from build123d import *

# Parameters (mm, degrees)
BOSS_EXTRUDE1_DEPTH = 150
SKETCH2_R           = 4.5
CUT_EXTRUDE2_DEPTH  = 12.5
SKETCH3_R           = 9.5
BOSS_EXTRUDE2_DEPTH = 55.5
SKETCH4_R           = 27.75
BOSS_EXTRUDE3_DEPTH = 2
SKETCH5_W           = 6
SKETCH5_H           = 35
BOSS_EXTRUDE4_DEPTH = 12


with BuildPart() as part:
    # Sketch1 → Boss-Extrude1 (new body)
    with BuildSketch(Plane(origin=(0, 0, 0), x_dir=(1, 0, 0), z_dir=(0, 1, 0))):
        with BuildLine():
            Line((-44.5, 55), (44.5, 55))
            ThreePointArc((44.5, 55), (51.924621202, 51.924621202), (55, 44.5))
            Line((55, 44.5), (55, -44.5))
            ThreePointArc((55, -44.5), (51.924621202, -51.924621202), (44.5, -55))
            Line((44.5, -55), (-44.5, -55))
            ThreePointArc((-44.5, -55), (-51.924621202, -51.924621202), (-55, -44.5))
            Line((-55, -44.5), (-55, 44.5))
            ThreePointArc((-55, 44.5), (-51.924621202, 51.924621202), (-44.5, 55))
        make_face()
    extrude(amount=BOSS_EXTRUDE1_DEPTH)

    # Sketch2 → Cut-Extrude2 (cut)
    with BuildSketch(Plane(origin=(0, 150, 0), x_dir=(1, 0, 0), z_dir=(0, 1, 0))):
        with Locations(Location((-44.5, 44.5, 0), (0, 0, 270))):
            Circle(SKETCH2_R)
        with Locations(Location((44.5, 44.5, 0), (0, 0, 270))):
            Circle(SKETCH2_R)
        with Locations(Location((-44.5, -44.5, 0), (0, 0, 270))):
            Circle(SKETCH2_R)
        with Locations(Location((44.5, -44.5, 0), (0, 0, 270))):
            Circle(SKETCH2_R)
    extrude(amount=-CUT_EXTRUDE2_DEPTH, mode=Mode.SUBTRACT)

    # Sketch3 → Boss-Extrude2 (add)
    with BuildSketch(Plane(origin=(0, 150, 0), x_dir=(1, 0, 0), z_dir=(0, 1, 0))):
        with Locations(Location((0, 0, 0), (0, 0, 270))):
            Circle(SKETCH3_R)
    extrude(amount=BOSS_EXTRUDE2_DEPTH)

    # Sketch4 → Boss-Extrude3 (add)
    with BuildSketch(Plane(origin=(0, 150, 0), x_dir=(1, 0, 0), z_dir=(0, 1, 0))):
        with Locations(Location((0, 0, 0), (0, 0, 270))):
            Circle(SKETCH4_R)
    extrude(amount=BOSS_EXTRUDE3_DEPTH)

    # Sketch5 → Boss-Extrude4 (add)
    with BuildSketch(Plane(origin=(0, 0, 0), x_dir=(0, 0, -1), z_dir=(1, 0, 0))):
        with Locations((0, 188)):
            Rectangle(SKETCH5_W, SKETCH5_H)
    extrude(amount=BOSS_EXTRUDE4_DEPTH)


solid = part.part
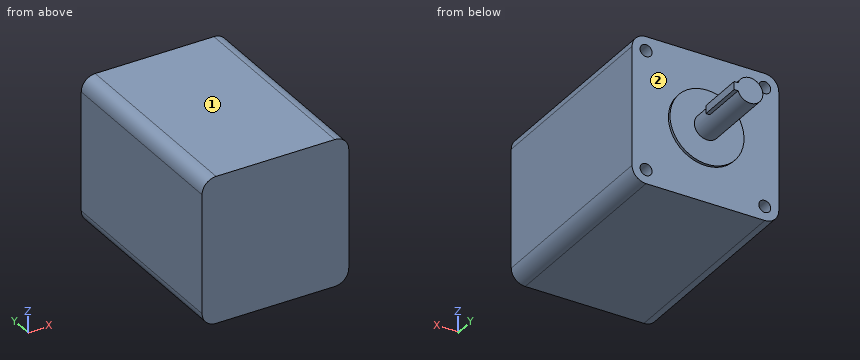
Read the model definition and answer for the solid it produces. Units are mm, in the model's axes. Face numbers are marked on the shaded views. A direction names the side the tool comes from. Coordinates: 2 decimals unless noted, no trailing zeros. Order: outer loops, then holes, each group sorted by start corner. A loop starts at its lowest first (then second) coordinate and runs counter-clockwise, first axis right, second up. Notation, with made-up numbers: (32, 5.25) -> (63, 5.25) arc R31 ccw to (63, 32.25) -> close; hole circle Ø4 at (34, -37.5). An arc over 180 degrees is marked (long way). Answer as a JSON object with one key per item and string values.
1) A cutting plane is placed at D-D, the plane z = 0. Determine the outline of the cut face in (x, y), plus the area to 3 significant figures.
Model answer:
{"outline": "(-55, 0) -> (55, 0) -> (55, 150) -> (27.75, 150) -> (27.75, 152) -> (9.5, 152) -> (9.5, 170.5) -> (12, 170.5) -> (12, 205.5) -> (-9.5, 205.5) -> (-9.5, 152) -> (-27.75, 152) -> (-27.75, 150) -> (-55, 150) -> close", "area": "17,700 mm²"}
2) A cutting plane is placed at C-C, the plane y = 156. Determine the outline of the cut face in (x, z).
Model answer:
{"outline": "circle Ø19 at (0, 0)"}
3) Each of these flat-tipped pins is pushed along its axis until it touches: pin 1 (3 mm diameter, centred on y = 179.5, z = -1, fed in from +X); pin 2 (1 mm diameter, centred on x = -16.5, z = -1, fed in from +Y); pin 3 (1 mm diameter, centred on x = 38, z = 23.5, fed in from +Y). Where does it stop, or does it pass through?
Model answer:
{"pin 1": "stops at x = 12", "pin 2": "stops at y = 152", "pin 3": "stops at y = 150"}
4) A cutting plane is placed at A-A, the plane x = 0. Determine the outline of the cut face in (y, z), plus the area to 3 significant figures.
Model answer:
{"outline": "(0, -55) -> (150, -55) -> (150, -27.75) -> (152, -27.75) -> (152, -9.5) -> (205.5, -9.5) -> (205.5, 9.5) -> (152, 9.5) -> (152, 27.75) -> (150, 27.75) -> (150, 55) -> (0, 55) -> close", "area": "17,600 mm²"}
5) A tool of negligible diameter and unlimited length cuts with its end or side. For the marked faces 1 and 2, from which of +Z, -Z, +X, -X, +Y, -Y can it reach the whole face along a straight path? Write none if from no direction.
Model answer:
{"face 1": "+Z, +X, -X, +Y, -Y", "face 2": "+Y"}
6) A cutting plane is placed at B-B, the plane z = 22. Determine the outline of the cut face in (x, y), plus the area to 3 significant figures.
Model answer:
{"outline": "(-55, 0) -> (55, 0) -> (55, 150) -> (16.91, 150) -> (16.91, 152) -> (-16.91, 152) -> (-16.91, 150) -> (-55, 150) -> close", "area": "16,600 mm²"}
7) Consider line 1 along X through (y, z) = (142.5, 44.5); line 2 along Z through (x, y) = (-44, 142); line 3 along Y through (x, z) = (-41, 28.5). Determine where each line is inside the solid, lowest interval first. Write a range as from..to.
Model answer:
{"line 1": "x = -55..-49, -40..40, 49..55", "line 2": "z = -55..-48.97, -40.03..40.03, 48.97..55", "line 3": "y = 0..150"}
